from build123d import *

# Parameters (mm, degrees)
PAD002_DEPTH    = 5
POCKET001_DEPTH = 41.001
SKETCH006_R     = 1.7
POCKET002_DEPTH = 41.001
POCKET003_DEPTH = 12
FILLET001_R     = 3
FILLET002_R     = 1


with BuildPart() as part:
    # Sketch004 → Pad002 (new body, symmetric)
    with BuildSketch(Plane.XY):
        with BuildLine():
            Line((0, 0), (0, 2.8))
            Line((0, 2.8), (9, 2.8))
            Line((9, 2.8), (9, 6))
            Line((9, 6), (0, 6))
            Line((0, 6), (0, 8.8))
            Line((0, 8.8), (9, 8.8))
            Line((9, 8.8), (9, 12))
            Line((9, 12), (0, 12))
            Line((0, 12), (0, 14.8))
            Line((0, 14.8), (9, 14.8))
            Line((9, 14.8), (9, 23.5))
            ThreePointArc((26.5, 41), (14.1256313292, 35.8743686708), (9, 23.5))
            Line((26.5, 41), (83, 41))
            Line((83, 41), (83, 30))
            Line((83, 30), (26.5, 30))
            ThreePointArc((26.5, 30), (21.9038059223, 28.0961940777), (20, 23.5))
            Line((20, 23.5), (20, 0))
            Line((20, 0), (0, 0))
        make_face()
    extrude(amount=PAD002_DEPTH, both=True)

    # Sketch005 (on Face18 of Pad002) → Pocket001 (cut, through all)
    with BuildSketch(Plane.XZ):
        with BuildLine():
            ThreePointArc((5, 5), (0, 0), (5, -5))
            Line((5, -6), (5, -5))
            Line((-1, -6), (5, -6))
            Line((-1, 6), (-1, -6))
            Line((5, 6), (-1, 6))
            Line((5, 6), (5, 5))
        make_face()
    extrude(amount=-POCKET001_DEPTH, mode=Mode.SUBTRACT)

    # Sketch006 (on Face2 of Pocket001) → Pocket002 (cut, through all)
    with BuildSketch(Plane.XZ):
        with Locations((3.5, 0)):
            Circle(SKETCH006_R)
    extrude(amount=-POCKET002_DEPTH, mode=Mode.SUBTRACT)

    # Sketch007 (on Face20 of Pocket002) → Revolution (revolve)
    with BuildSketch(Plane.YZ.offset(78)):
        Polygon((21.3046738147, -3.0383206522), (34.6684285365, 2.2847238185), (35.5, 0), (21.9887141013, -4.9177058938), align=None)
    revolve(axis=Axis((78, 4.1527111346, -11.4094800719), (0, 0.9396926208, 0.3420201433)))

    # Sketch008 (on Face20 of Revolution) → Pocket003 (cut)
    with BuildSketch(Plane.YZ.offset(83)):
        Polygon((30, -4.3490166725), (41, 2.0018362885), (41, -5), (30, -5), align=None)
    extrude(amount=-POCKET003_DEPTH, mode=Mode.SUBTRACT)

    # Fillet001
    fillet001_edges = [part.edges().sort_by_distance(p)[0] for p in [
        (71, 35.5, -1.17359),
    ]]
    fillet(fillet001_edges, radius=FILLET001_R)

    # Fillet002
    fillet002_edges = [part.edges().sort_by_distance(p)[0] for p in [
        (83, 30, 0.325492),
        (83, 35.5, 5),
        (83, 41, 3.500918),
        (83, 35.5, -1.17359),
    ]]
    fillet(fillet002_edges, radius=FILLET002_R)


solid = part.part
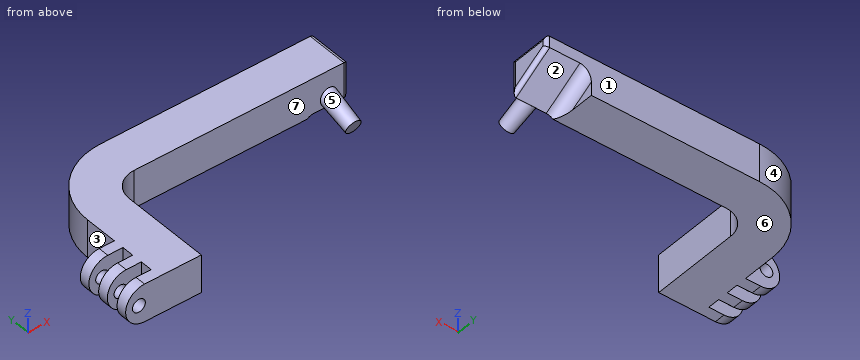
Build history of the part. All positions in model axes, mm. Face numbers are marked on the shaded views. A direction names the side the tool comes from. Round coordinates to 2 decimals unless told otherwise and drop trailing zeros. Write each loop counter-clockwise with the first axis right and the second up, starting at its lowest first coordinate (ties: lowest second). Pieces come first, ordered by that corner, then holes. Notation, with made-up numbers: M -14,29 L -4,29 A18 cw -4,39 Z; hole C 18,59.5 d9. An arc over 180 degrees is marked long. Answer in a Markdown table with one row per item.
1. Which spindle directions (+Z, -Z, +X, -X, +Y, -Y) get a long thin tool onto all of the face, cutting with end or side? Do the marked faces 1, 2 and 3. Say none if no direction does.
Geometry check:
| item | result |
|---|---|
| face 1 | +Z, -Z, +X, -X, +Y |
| face 2 | -Z, +X, +Y |
| face 3 | +Z, -Z, -X, +Y |
2. Saw through at A-A (x = 3.5). List the corners of the cut face in (y, z).
Geometry check:
| item | result |
|---|---|
| outline | M 0,-4.77 L 2.8,-4.77 L 2.8,-1.7 L 0,-1.7 Z; M 0,1.7 L 2.8,1.7 L 2.8,4.77 L 0,4.77 Z; M 6,-4.77 L 8.8,-4.77 L 8.8,-1.7 L 6,-1.7 Z; M 6,1.7 L 8.8,1.7 L 8.8,4.77 L 6,4.77 Z; M 12,-4.77 L 14.8,-4.77 L 14.8,-1.7 L 12,-1.7 Z; M 12,1.7 L 14.8,1.7 L 14.8,4.77 L 12,4.77 Z |
3. Saw through at B-B (x = 46). List the corners of the cut face in (y, z).
Geometry check:
| item | result |
|---|---|
| outline | M 30,-5 L 41,-5 L 41,5 L 30,5 Z |
4. Flat gauge pins, fed straight in: P1, Ø2, axis at x = 17.5, z = -3, coming from the -Y side; P2, Ø4.5, axis at x = 6, z = -1, coming from the +Y side; P3, Ø3, axis at y = 12.5, z = -2, coming from the +X side; P4, Ø6, axis at y = 25.5, z = -1, coming from the +X side. Where does each tip first touch, or does it go through?
Geometry check:
| item | result |
|---|---|
| P1 | y = 0 |
| P2 | y = 14.8 |
| P3 | x = 20 |
| P4 | x = 80.19 |
5. Probe L1, parallel to Y at x = 4.5, z = 2; L2, parallel to Y at x = 70.5, z = 3.75; L3, parallel to Z at x = 48, y = 38. List the from-to ranges inside material, lowest first. Write a range as [from, to].
Geometry check:
| item | result |
|---|---|
| L1 | [0, 2.8], [6, 8.8], [12, 14.8] |
| L2 | [30, 41] |
| L3 | [-5, 5] |
6. Mould opens along X. For the marked faces 4, 5, 6 and 7 say: +X half, -X half, draft (parallel to the pull), parting line (faces both ways), or undercut.
Geometry check:
| item | result |
|---|---|
| face 4 | -X half |
| face 5 | undercut |
| face 6 | draft |
| face 7 | undercut |
